Read the model definition and answer for the solid it produces. Units are mm, in the model's axes. A direction names the side the tool comes from. Coordinates: 2 decimals unless noted, no trailing zeros. Loops run counter-clockwise (first coordinate to the right, second up) from the corner with the lowest first, then second, coordinate; pieces in that order, holes last. Notation, with made-up numbers: (4, 16.5) -> (61, 16.5) arc R31 cw to (61, 41.5) -> close; hole circle Ø2 at (64.5, -6). An arc over 180 degrees is marked (long way). Answer as CSV lines item,"result".
```python
from build123d import *

# Parameters (mm, degrees)
F0_R     = 3.81
F1_DEPTH = 19.05
F2_R     = 3.81
F3_R     = 1.27


with BuildPart() as f1:
    # F0 (on Front) → F1 (new body)
    with BuildSketch(Plane.XZ):
        Polygon((114.3, 65.991136), (76.2, 131.982272), (65.991136, 114.3), (0, 152.4), (0, 131.982272), (-76.2, 131.982272), (-65.991136, 114.3), (-131.982272, 76.2), (-114.3, 65.991136), (-152.4, 0), (-131.982272, 0), (-131.982272, -76.2), (-114.3, -65.991136), (-76.2, -131.982272), (-65.991136, -114.3), (0, -152.4), (0, -131.982272), (76.2, -131.982272), (65.991136, -114.3), (131.982272, -76.2), (114.3, -65.991136), (152.4, 0), (131.982272, 0), (131.982272, 76.2), align=None)
        with Locations((0, -35.56)):
            Circle(F0_R, mode=Mode.SUBTRACT)
        with Locations((-35.56, 0)):
            Circle(F0_R, mode=Mode.SUBTRACT)
        with BuildLine():
            ThreePointArc((-12.7, -19.05), (-15.875, -20.365128), (-19.05, -19.05))
            ThreePointArc((-19.05, -19.05), (-20.365128, -15.875), (-19.05, -12.7))
            Line((-19.05, -12.7), (-19.05, 12.7))
            ThreePointArc((-19.05, 12.7), (-20.365128, 15.875), (-19.05, 19.05))
            ThreePointArc((-19.05, 19.05), (-15.875, 20.365128), (-12.7, 19.05))
            Line((-12.7, 19.05), (12.7, 19.05))
            ThreePointArc((12.7, 19.05), (15.875, 20.365128), (19.05, 19.05))
            ThreePointArc((19.05, 19.05), (20.023337, 17.593298), (20.365128, 15.875))
            ThreePointArc((20.365128, 15.875), (20.023337, 14.156702), (19.05, 12.7))
            Line((19.05, 12.7), (19.05, -12.7))
            ThreePointArc((19.05, -12.7), (20.023337, -14.156702), (20.365128, -15.875))
            ThreePointArc((20.365128, -15.875), (20.023337, -17.593298), (19.05, -19.05))
            ThreePointArc((19.05, -19.05), (15.875, -20.365128), (12.7, -19.05))
            Line((12.7, -19.05), (-12.7, -19.05))
        make_face(mode=Mode.SUBTRACT)
        with Locations((35.56, 0)):
            Circle(F0_R, mode=Mode.SUBTRACT)
        with Locations((0, 35.56)):
            Circle(F0_R, mode=Mode.SUBTRACT)
    extrude(amount=F1_DEPTH)

    # F2
    f2_edges = [f1.edges().sort_by_distance(p)[0] for p in [
        (65.991136, -9.525, 114.3),
        (114.3, -9.525, 65.991136),
        (131.982272, -9.525, 0),
        (114.3, -9.525, -65.991136),
        (65.991136, -9.525, -114.3),
        (0, -9.525, -131.982272),
        (-65.991136, -9.525, -114.3),
        (-114.3, -9.525, -65.991136),
        (-131.982272, -9.525, 0),
        (-114.3, -9.525, 65.991136),
        (-65.991136, -9.525, 114.3),
        (0, -9.525, 131.982272),
    ]]
    fillet(f2_edges, radius=F2_R)

    # F3
    f3_edges = [f1.edges().sort_by_distance(p)[0] for p in [
        (0, -9.525, 152.4),
        (76.2, -9.525, 131.982272),
        (131.982272, -9.525, 76.2),
        (152.4, -9.525, 0),
        (131.982272, -9.525, -76.2),
        (76.2, -9.525, -131.982272),
        (0, -9.525, -152.4),
        (-76.2, -9.525, -131.982272),
        (-131.982272, -9.525, -76.2),
        (-152.4, -9.525, 0),
        (-131.982272, -9.525, 76.2),
        (-76.2, -9.525, 131.982272),
    ]]
    fillet(f3_edges, radius=F3_R)


solid = f1.part
```
Q1. For faces 1 (the face through (71.55, -9.39, -123.93)), 2 (the face through (123.93, -9.39, 71.55)), 3 (the face through (131.982, -9, 38)), 4 (the face through (0, -9, -143)), 5 (the face through (-143, -9, 0)), determine the directions among +Z, -Z, +X, -X, +Y, -Y from which every point of the face is accessible in a straight line to the end or side of a thin tool.
Results:
face 1,"+X, +Y, -Y"
face 2,"+Z, +Y, -Y"
face 3,"+Z, +X, +Y, -Y"
face 4,"-Z, +X, +Y, -Y"
face 5,"-Z, -X, +Y, -Y"
Q2. Find the intervals of material crossed by probe 1 along Z at (x, y) = (35.56, -11.5); probe 2 along Z at (x, y) = (-35.56, -10); probe 3 along Z at (x, y) = (64, -1.75), in increasing order. Write a range as [from, to].
Results:
probe 1,"z = [-131.98, -3.81], [3.81, 131.87]"
probe 2,"z = [-131.87, -3.81], [3.81, 131.98]"
probe 3,"z = [-131.98, 115.74]"
Q3. A cutting plane is placed at C-C, the plane y = -16. Give the number of separate pieces and of enclosed holes in the cut face, and give its area (3 significant figures).
Results:
separate pieces,"1"
enclosed holes,"5"
area,"58,700 mm²"
Q4. For a pull along X with two mould halves and no side action, classify faces 6 (the face through (123.93, -9.39, -71.55)), 7 (the face through (-71.55, -9.39, -123.93)), 8 (the face through (143, -9, 0)) as pulls with the +X half, pulls with the -X half, needs draft (parallel to the pull), parting line crosses it, or undercut.
Results:
face 6,"pulls with the +X half"
face 7,"undercut"
face 8,"needs draft"
Q5. Given pin 1 Ø1.5 at (y, z) = (-8.5, 63.5) entering from +X; pin 2 Ø1 at (y, z) = (-11.5, -112) entering from -X; pin 3 Ø5 at (y, z) = (-13.5, 107.5) entering from +X; pin 4 Ø9.5 at (x, y) = (-3, -13) entering from -Z, each flat-ended and moving along its own axis, determine where each tip first touches the part or whether it passes through.
Results:
pin 1,"stops at x = 131.98"
pin 2,"stops at x = -88.03"
pin 3,"stops at x = 91.78"
pin 4,"stops at z = -151.47"
Q6. A cutting plane is placed at D-D, the plane z = -87. Write down the section's boundary in (x, y).
Results:
outline,"(-102.17, -19.05) -> (113.28, -19.05) -> (113.28, 0) -> (-102.17, 0) -> close"
Q7. A cutting plane is placed at A-A, the plane x = -35.56. Write down the section's boundary in (y, z), and give its area (3 significant figures).
Results:
outline,"(-19.05, -131.87) -> (0, -131.87) -> (0, -3.81) -> (-19.05, -3.81) -> close; (-19.05, 3.81) -> (0, 3.81) -> (0, 131.98) -> (-19.05, 131.98) -> close"
area,"4,880 mm²"
Q8. A cutting plane is placed at B-B, the plane z = 35.56. Write down the section's boundary in (x, y), and give its area (3 significant figures).
Results:
outline,"(-131.87, -19.05) -> (-3.81, -19.05) -> (-3.81, 0) -> (-131.87, 0) -> close; (3.81, -19.05) -> (131.98, -19.05) -> (131.98, 0) -> (3.81, 0) -> close"
area,"4,880 mm²"
